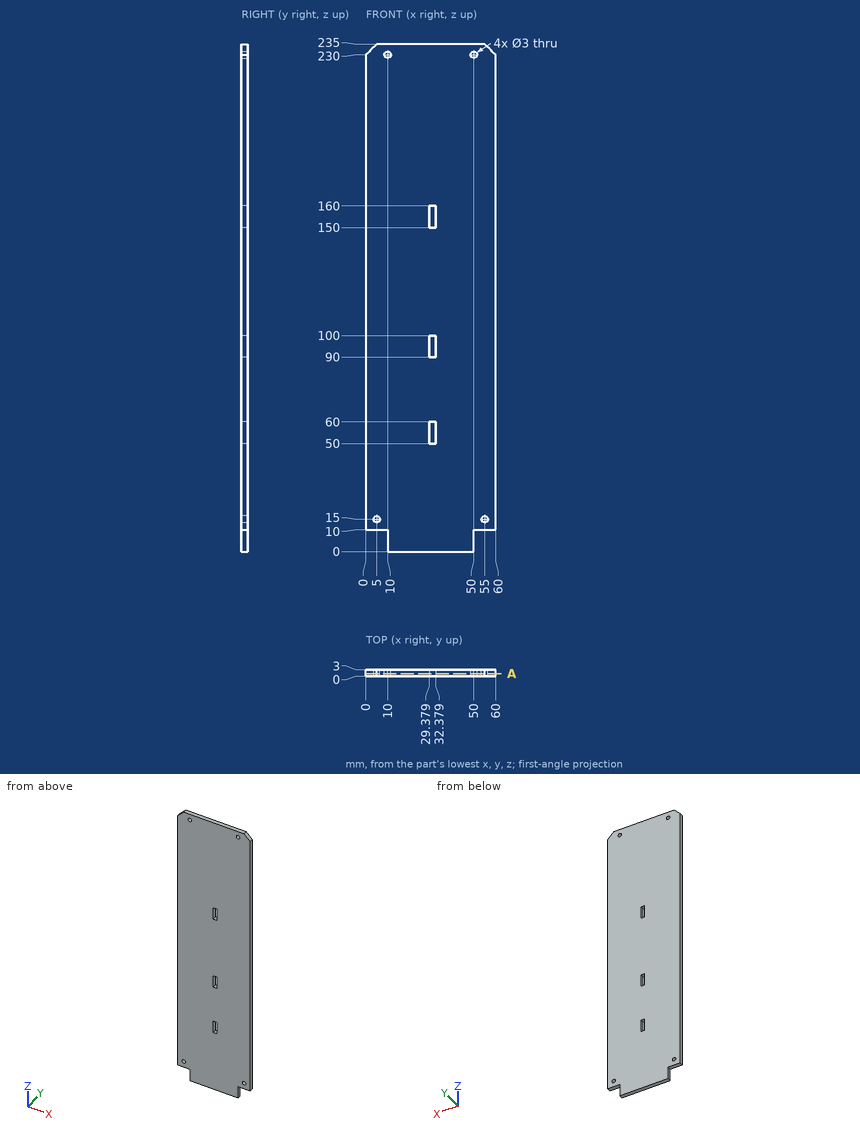
Here's the drawing with two shaded views (mm, measured from the low corner). I have some questions. Coordinates: 2 decimals unless noted, no trailing zeros. Loops run counter-clockwise (first coordinate to the right, second up) from the corner with the lowest first, then second, coordinate; pieces in that order, holes last. Notation, with made-up numbers: (69.25, -14) -> (115.25, -14) arc R23 cw to (115.25, 13) -> close; hole circle Ø7 at (-36, 41). An arc over 180 degrees is marked (long way). Answer in a Markdown table with one row per item.
(1) Imagine slicing it at A-A (y = 1.1). List the corners of the cut face in (x, z) for me, plus the area to 3 significant figures.
Results found:
| item | result |
|---|---|
| outline | (0, 10) -> (10, 10) -> (10, 0) -> (50, 0) -> (50, 10) -> (60, 10) -> (60, 230) -> (55, 235) -> (5, 235) -> (0, 230) -> close; hole circle Ø3 at (5, 15); hole circle Ø3 at (10, 230); hole (29.38, 50) -> (32.38, 50) -> (32.38, 60) -> (29.38, 60) -> close; hole (29.38, 90) -> (32.38, 90) -> (32.38, 100) -> (29.38, 100) -> close; hole (29.38, 150) -> (32.38, 150) -> (32.38, 160) -> (29.38, 160) -> close; hole circle Ø3 at (50, 230); hole circle Ø3 at (55, 15) |
| area | 13,800 mm^2 |
(2) If I drill on probe 1 along X at (y, z) = (2.05, 230); probe 2 along X at (y, z) = (0.65, 99); probe 3 along X at (y, z) = (0.8, 15), over which ranges is the centre line in solid material (lowest first)?
Results found:
| item | result |
|---|---|
| probe 1 | x = 0 to 8.5, 11.5 to 48.5, 51.5 to 60 |
| probe 2 | x = 0 to 29.38, 32.38 to 60 |
| probe 3 | x = 0 to 3.5, 6.5 to 53.5, 56.5 to 60 |
(3) Will these pins go through, and if not, where does the flat tip stop? pin 1 Ø1.5 at (x, y) = (7, 1.5) entering from -Z; pin 2 Ø1.5 at (y, z) = (1.5, 4.5) entering from +X; pin 3 Ø2.5 at (x, z) = (5, 15) entering from +Y.
Results found:
| item | result |
|---|---|
| pin 1 | stops at z = 10 |
| pin 2 | stops at x = 50 |
| pin 3 | passes through |
